Answer from the drawing. Dimensions are ordinates in mm from the lowest x, y and z of the part. Give positions to 0.01 mm unless a question says otherwise; leave off trailing zeros. Order: outer loops, then holes, each group sorted by start corner. A loop starts at its lowest first (then second) coordinate and runs counter-clockwise, first axis right, second up.
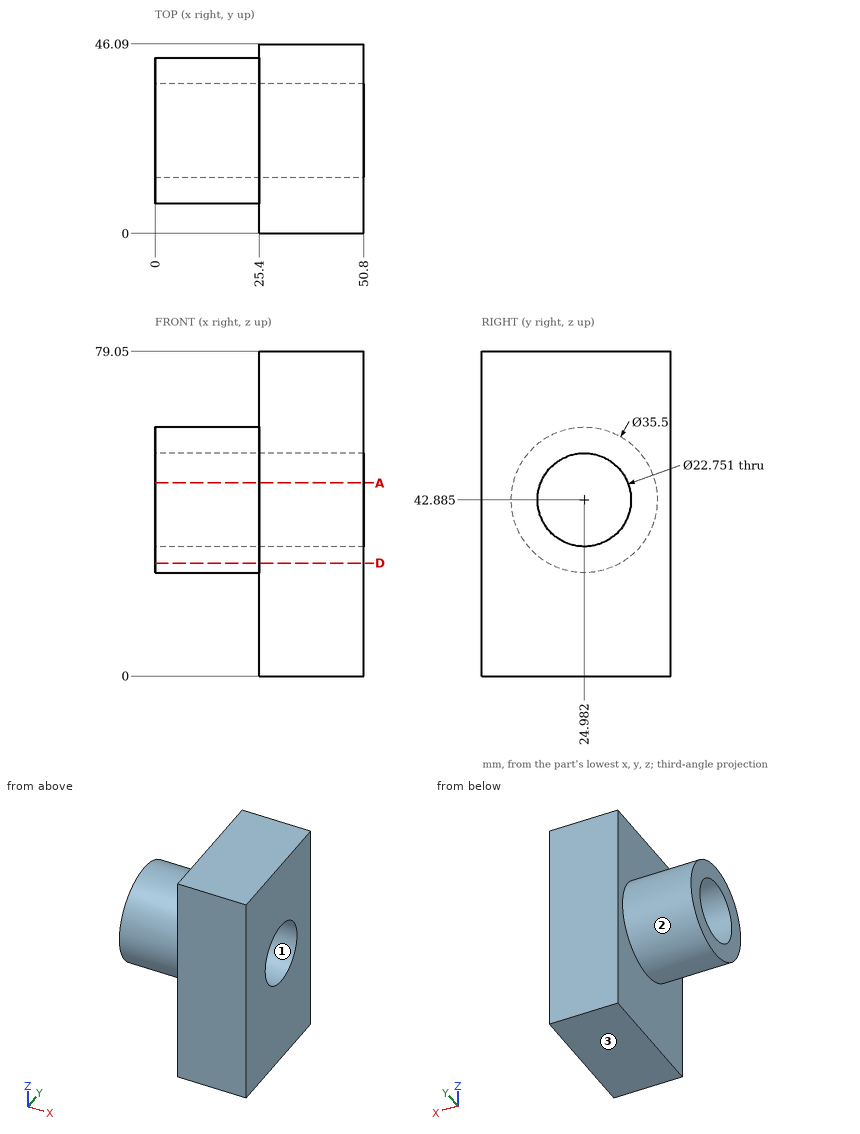
1) Consider L1, parallel to X at y = 4, z = 68; L2, parallel to Z at x = 36, y = 25; L3, parallel to Z at x = 20, y = 29 (1 decimal). Determine where each line is inside the solid, lowest interval first.
Final values:
L1: x = 25.4 to 50.8
L2: z = 0 to 31.51, 54.26 to 79.05
L3: z = 25.6 to 32.2, 53.5 to 60.2
2) Given pin 1 (4 mm diameter, centred on y = 24, z = 24.5, fed in from -X); pin 2 (4 mm diameter, centred on x = 21, y = 38, fed in from -Z); pin 3 (18 mm diameter, centred on y = 24.98, z = 42.89, fed in from +X), each flat-ended and moving along its own axis, determine where each tip first touches the part or whether it passes through.
Final values:
pin 1: stops at x = 0
pin 2: stops at z = 28.97
pin 3: passes through
3) The part is cut by section A-A on z = 47. Determine the outline of the cut face in (x, y) (1 decimal).
Final values:
outline: (0, 7.7) - (25.4, 7.7) - (25.4, 0) - (50.8, 0) - (50.8, 14.4) - (0, 14.4) - close; (0, 35.6) - (50.8, 35.6) - (50.8, 46.1) - (25.4, 46.1) - (25.4, 42.2) - (0, 42.2) - close
4) For a pull along Y with two mould halves and no side action, classify the marked faces 1, 2 and 3 as released by +Y, released by -Y, zero draft, split by the parting line, or undercut.
Final values:
face 1: undercut
face 2: split by the parting line
face 3: zero draft
5) The part is cut by section D-D on z = 27.5. Determine the outline of the cut face in (x, y), and give its area (3 significant figures).
Final values:
outline: (0, 16.13) - (25.4, 16.13) - (25.4, 0) - (50.8, 0) - (50.8, 46.09) - (25.4, 46.09) - (25.4, 33.83) - (0, 33.83) - close
area: 1,620 mm2
